Design review of the part built by this model. Coordinates are the model's own, in mm. Face numbers are marked on the shaded views. A direction names the side the tool comes from. Coordinates: 2 decimals unless noted, no trailing zeros. Loops run counter-clockwise (first coordinate to the right, second up) from the corner with the lowest first, then second, coordinate; pieces in that order, holes last. Notation, with made-up numbers: (-11.5, -21) -> (1.5, -21) arc R7 cw to (1.5, -13) -> close; hole circle Ø5 at (-20, -23.75). An arc over 180 degrees is marked (long way). Use a Markdown table: item, result. Add a question column.
Q1. Draft analysis for pull direction X (two halves, no side actions). For the marked faces 1, 2 and 3, state which applies: pulls with the +X half, pulls with the -X half, needs draft (parallel to the pull), parting line crosses it, or undercut.
Q2. Clearance check with flat-ended pins moving along their axes: pin 1 Ø4 at (x, z) = (-8, 2) entering from +Y; pin 2 Ø9 at (x, z) = (8.5, 2.5) entering from -Y; pin 3 Ø3 at (x, z) = (-3.5, 0.5) entering from -Y (3 decimals); pin 4 Ø0.8 at (x, z) = (17.5, 8) entering from +Y. State where each tip first meets the part, or that it passes through.
Q3. Take a section at B-B on z = 0. Count the separate pieces of the cut face and the enclosed holes in it, plus the area to 3 significant figures.
Q4. Take a section at C-C on y = -12.5. Write out the cut boundary in (x, z).
Q5. Take a section at A-A on y = 2.5. Write out the cut boundary in (x, z) (1 decimal).
Q6. For the marked faces 4, 5 and 6, list the 3-axis set-ups (+Z, -Z, +X, -X, +Y, -Y) from which the entire face can be reached by the end or side of a thin tool; tool diameter is ignored.
Q7. For probe 1 along Z at (x, y) = (16, -19.5); probe 2 along X at (y, z) = (3.4, 0) (1 decimal); probe 3 along Z at (x, y) = (-4.5, -17), list the stretches that pass through material, from the lowest coordinate up.
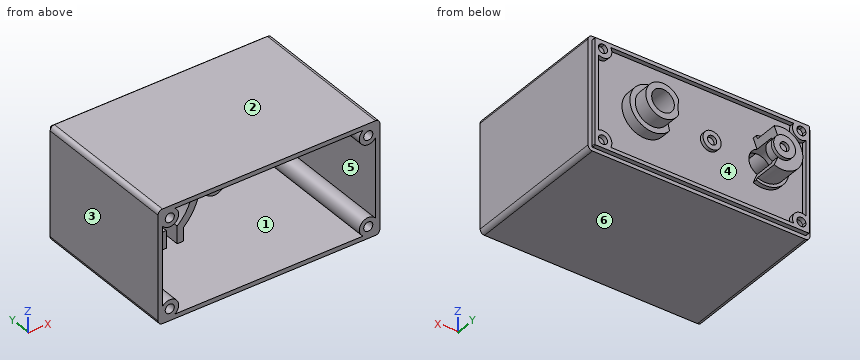
from build123d import *

# Parameters (mm, degrees)
SKETCH1_R                       = 2.3495
SKETCH1_R_2                     = 1.9812
EXTRUDE1_DEPTH                  = 1.190625
SKETCH6_R                       = 1.5875
SKETCH6_R_2                     = 0.79375
EXTRUDE3_DEPTH                  = 0.6096
SKETCH7_R                       = 3
SKETCH7_R_2                     = 1.9812
EXTRUDE4_DEPTH                  = 4.445
SKETCH16_R                      = 3.937
SKETCH16_R_2                    = 3
EXTRUDE11_DEPTH                 = 1.905
CUT_EXTRUDE1_REACH              = 24.444
SKETCH11_R                      = 7.874
SKETCH11_R_2                    = 6.604
EXTRUDE6_DEPTH                  = 4.572
SKETCH10_W                      = 37.211
SKETCH10_H                      = 18.161
EXTRUDE5_DEPTH                  = 25.90546
SKETCH13_W                      = 1.143
SKETCH13_H                      = 3.048
EXTRUDE8_DEPTH                  = 10.795
EXTRUDE9_START                  = -1.952625
SKETCH14_R                      = 0.79375
EXTRUDE9_DEPTH                  = 26.66746
SKETCH23_R                      = 0.79375
CUT_EXTRUDE2_DEPTH              = 1.190625
CUT_EXTRUDE3_REACH              = 39.594
MIRROR2_START                   = -1.952625
MIRROR2_COPY_1_SKETCH_R         = 0.79375
MIRROR2_COPY_1_DEPTH            = 26.66746
SKETCH18_W                      = 36.195
SKETCH18_H                      = 17.145
EXTRUDE12_DEPTH                 = 0.762
SKETCH19_R                      = 2.54
EXTRUDE13_DEPTH                 = 1.905
EXTRUDE14_DEPTH                 = 5.588
F_1_64_TAPPED_HOLE1_D           = 1.5113
F_1_64_TAPPED_HOLE1_DEPTH       = 5.588
F_1_64_TAPPED_HOLE1_CBORE_D     = 1.8542
F_1_64_TAPPED_HOLE1_CBORE_DEPTH = 3.7084


with BuildPart() as part:
    # Sketch1 → Extrude1 (new body)
    with BuildSketch(Plane(origin=(0, 0, 0), x_dir=(1, 0, 0), z_dir=(0, 1, 0))):
        with BuildLine():
            Line((-18.6055, 9.8425), (18.6055, 9.8425))
            ThreePointArc((18.6055, 9.8425), (19.144315367, 9.619315367), (19.3675, 9.0805))
            Line((19.3675, 9.0805), (19.3675, -9.0805))
            ThreePointArc((19.3675, -9.0805), (19.144315367, -9.619315367), (18.6055, -9.8425))
            Line((18.6055, -9.8425), (-18.6055, -9.8425))
            ThreePointArc((-18.6055, -9.8425), (-19.144315367, -9.619315367), (-19.3675, -9.0805))
            Line((-19.3675, -9.0805), (-19.3675, 9.0805))
            ThreePointArc((-19.3675, 9.0805), (-19.144315367, 9.619315367), (-18.6055, 9.8425))
        make_face()
        with Locations(Location((-11.049, 0, 0), (0, 0, 90))):
            Circle(SKETCH1_R, mode=Mode.SUBTRACT)
        with Locations(Location((9.525, 0, 0), (0, 0, 90))):
            Circle(SKETCH1_R_2, mode=Mode.SUBTRACT)
    extrude(amount=EXTRUDE1_DEPTH)

    # Sketch6 → Extrude3 (add)
    with BuildSketch(Plane(origin=(0, 1.190625, 0), x_dir=(-1, 0, 0), z_dir=(0, 1, 0))):
        with Locations(Location((1.8415, 0, 0), (0, 0, 270))):
            Circle(SKETCH6_R)
        with Locations(Location((1.8415, 0, 0), (0, 0, 90))):
            Circle(SKETCH6_R_2, mode=Mode.SUBTRACT)
    extrude(amount=EXTRUDE3_DEPTH)

    # Sketch7 → Extrude4 (add)
    with BuildSketch(Plane(origin=(0, 1.190625, 0), x_dir=(-1, 0, 0), z_dir=(0, 1, 0))):
        with Locations(Location((-9.525, 0, 0), (0, 0, 270))):
            Circle(SKETCH7_R)
        with Locations(Location((-9.525, 0, 0), (0, 0, 270))):
            Circle(SKETCH7_R_2, mode=Mode.SUBTRACT)
    extrude(amount=EXTRUDE4_DEPTH)

    # Sketch16 → Extrude11 (add)
    with BuildSketch(Plane(origin=(0, 1.190625, 0), x_dir=(-1, 0, 0), z_dir=(0, 1, 0))):
        with Locations(Location((-9.525, 0, 0), (0, 0, 270))):
            Circle(SKETCH16_R)
        with Locations(Location((-9.525, 0, 0), (0, 0, 90))):
            Circle(SKETCH16_R_2, mode=Mode.SUBTRACT)
    extrude(amount=EXTRUDE11_DEPTH)

    # Cut-Extrude1: up to this face of the body (flat: up to its plane)
    cut_extrude1_end = Plane(part.part.faces().sort_by_distance((0, 1.190625, -9.408000351))[0])
    # Sketch17 → Cut-Extrude1 (cut, up to the picked face)
    with BuildSketch(Plane(origin=(0, 5.635625, 0), x_dir=(-1, 0, 0), z_dir=(0, 1, 0)), mode=Mode.PRIVATE) as cut_extrude1_sk1:
        with BuildLine():
            ThreePointArc((-6.516949302, 2.54), (-6.894361419, 0), (-6.516949302, -2.54))
            ThreePointArc((-6.516949302, -2.54), (-5.588, 0), (-6.516949302, 2.54))
        make_face()
    cut_extrude1_tool1 = split(extrude(cut_extrude1_sk1.sketch, amount=-CUT_EXTRUDE1_REACH, mode=Mode.PRIVATE), bisect_by=cut_extrude1_end, keep=Keep.BOTH, mode=Mode.PRIVATE)
    add(cut_extrude1_tool1.solids().sort_by(Axis((6.291228, 5.635625, 0), (0, -1, 0)))[0], mode=Mode.SUBTRACT)

    # Sketch11 → Extrude6 (add)
    with BuildSketch(Plane.XZ):
        with Locations(Location((9.525, 0, 0), (0, 0, 270))):
            Circle(SKETCH11_R)
        with Locations(Location((9.525, 0, 0), (0, 0, 270))):
            Circle(SKETCH11_R_2, mode=Mode.SUBTRACT)
    extrude(amount=EXTRUDE6_DEPTH)

    # Sketch10 → Extrude5 (add)
    with BuildSketch(Plane.XZ.offset(-1.190625)):
        with BuildLine():
            Line((-19.3675, 9.0805), (-19.3675, -9.0805))
            ThreePointArc((-19.3675, -9.0805), (-19.144315367, -9.619315367), (-18.6055, -9.8425))
            Line((-18.6055, -9.8425), (18.6055, -9.8425))
            ThreePointArc((18.6055, -9.8425), (19.144315367, -9.619315367), (19.3675, -9.0805))
            Line((19.3675, -9.0805), (19.3675, 9.0805))
            ThreePointArc((19.3675, 9.0805), (19.144315367, 9.619315367), (18.6055, 9.8425))
            Line((18.6055, 9.8425), (-18.6055, 9.8425))
            ThreePointArc((-18.6055, 9.8425), (-19.144315367, 9.619315367), (-19.3675, 9.0805))
        make_face()
        Rectangle(SKETCH10_W, SKETCH10_H, mode=Mode.SUBTRACT)
    extrude(amount=EXTRUDE5_DEPTH)

    # Sketch13 → Extrude8 (add)
    with BuildSketch(Plane.XZ):
        with BuildLine():
            Line((-5.9055, 6.0325), (-5.9055, 9.0805))
            Line((-5.9055, 9.0805), (-4.7625, 9.0805))
            Line((-4.7625, 9.0805), (-4.7625, 6.713831938))
            ThreePointArc((-4.7625, 6.713831938), (-1.851412189, 0), (-4.7625, -6.713831938))
            Line((-4.7625, -6.713831938), (-4.7625, -9.0805))
            Line((-4.7625, -9.0805), (-5.9055, -9.0805))
            Line((-5.9055, -9.0805), (-5.9055, -6.0325))
            ThreePointArc((-5.9055, -6.0325), (-3.121412189, 0), (-5.9055, 6.0325))
        make_face()
        with Locations((-8.382, 7.5565)):
            Rectangle(SKETCH13_W, SKETCH13_H)
        with Locations((-13.335, 7.5565)):
            Rectangle(SKETCH13_W, SKETCH13_H)
        with Locations((-13.335, -7.5565)):
            Rectangle(SKETCH13_W, SKETCH13_H)
        with Locations((-8.382, -7.5565)):
            Rectangle(SKETCH13_W, SKETCH13_H)
    extrude(amount=EXTRUDE8_DEPTH)

    # Sketch14 → Extrude9 (add)
    with BuildSketch(Plane.XZ.offset(EXTRUDE9_START)):
        with BuildLine():
            Line((-18.6055, -9.0805), (-18.6055, -6.911913297))
            ThreePointArc((-18.6055, -6.911913297), (-16.235418625, -6.710418625), (-16.436913297, -9.0805))
            Line((-16.436913297, -9.0805), (-18.6055, -9.0805))
        make_face()
        with Locations(Location((-17.3355, -7.8105, 0), (0, 0, 270))):
            Circle(SKETCH14_R, mode=Mode.SUBTRACT)
    extrude9 = extrude(amount=EXTRUDE9_DEPTH)

    # Sketch23 → Cut-Extrude2 (cut)
    with BuildSketch(Plane(origin=(0, 1.190625, 0), x_dir=(-1, 0, 0), z_dir=(0, 1, 0))):
        with Locations(Location((17.3355, -7.8105, 0), (0, 0, 270))):
            Circle(SKETCH23_R)
    extrude(amount=-CUT_EXTRUDE2_DEPTH, mode=Mode.SUBTRACT)

    # Sketch9 → Revolve1 (revolve)
    with BuildSketch(Plane.XY, mode=Mode.PRIVATE) as revolve1_sk:
        Polygon((-12.954, 5.965825), (-12.954, 6.550025), (-11.84275, 6.550025), (-11.84275, 5.965825), (-11.049, 5.965825), (-11.049, 4.645025), (-13.3985, 4.645025), (-13.3985, 1.190625), (-15.1765, 1.190625), (-15.1765, 1.952625), (-14.6685, 1.952625), (-14.6685, 5.965825), align=None)
    revolve(revolve1_sk.sketch.rotate(Axis((-11.049, 0, 0), (0, 1, 0)), 270), axis=Axis((-11.049, 0, 0), (0, 1, 0)))

    # Cut-Extrude3: up to this face of the body (flat: up to its plane)
    cut_extrude3_end = Plane(part.part.faces().sort_by_distance((-1.8415, 1.190625, 0))[0])
    # Sketch24 → Cut-Extrude3 (cut, up to the picked face)
    with BuildSketch(Plane(origin=(0, 5.965825, 0), x_dir=(-1, 0, 0), z_dir=(0, 1, 0)), mode=Mode.PRIVATE) as cut_extrude3_sk1:
        with BuildLine():
            Line((10.316307692, 1.758461538), (9.4615, 3.81))
            ThreePointArc((9.4615, 3.81), (6.9215, 0), (9.4615, -3.81))
            Line((9.4615, -3.81), (10.316307692, -1.758461538))
            ThreePointArc((10.316307692, -1.758461538), (9.144, 0), (10.316307692, 1.758461538))
        make_face()
    cut_extrude3_tool1 = split(extrude(cut_extrude3_sk1.sketch, amount=-CUT_EXTRUDE3_REACH, mode=Mode.PRIVATE), bisect_by=cut_extrude3_end, keep=Keep.BOTH, mode=Mode.PRIVATE)
    add(cut_extrude3_tool1.solids().sort_by(Axis((-8.574349, 5.965825, 0), (0, -1, 0)))[0], mode=Mode.SUBTRACT)

    # Mirror1: Extrude9 across plane
    add(extrude9.mirror(Plane(origin=(0, 0, 0), x_dir=(0, 0, 1), z_dir=(1, 0, 0))))

    # Mirror2: Extrude9 across plane
    add(extrude9.mirror(Plane.XY))

    # Mirror2 copy 1 sketch → Mirror2 copy 1 (add)
    with BuildSketch(Plane(origin=(0, 0, 0), x_dir=(-1, 0, 0), z_dir=(0, -1, 0)).offset(MIRROR2_START)):
        with BuildLine():
            Line((-18.6055, -9.0805), (-18.6055, -6.911913297))
            ThreePointArc((-18.6055, -6.911913297), (-16.235418625, -6.710418625), (-16.436913297, -9.0805))
            Line((-16.436913297, -9.0805), (-18.6055, -9.0805))
        make_face()
        with Locations(Location((-17.3355, -7.8105, 0), (0, 0, 270))):
            Circle(MIRROR2_COPY_1_SKETCH_R, mode=Mode.SUBTRACT)
    extrude(amount=MIRROR2_COPY_1_DEPTH)

    # Sketch18 → Extrude12 (add)
    with BuildSketch(Plane(origin=(0, 1.952625, 0), x_dir=(-1, 0, 0), z_dir=(0, 1, 0))):
        with BuildLine():
            Line((18.6055, 9.2075), (-18.6055, 9.2075))
            ThreePointArc((-18.6055, 9.2075), (-18.695302561, 9.170302561), (-18.7325, 9.0805))
            Line((-18.7325, 9.0805), (-18.7325, -9.0805))
            ThreePointArc((-18.7325, -9.0805), (-18.695302561, -9.170302561), (-18.6055, -9.2075))
            Line((-18.6055, -9.2075), (18.6055, -9.2075))
            ThreePointArc((18.6055, -9.2075), (18.695302561, -9.170302561), (18.7325, -9.0805))
            Line((18.7325, -9.0805), (18.7325, 9.0805))
            ThreePointArc((18.7325, 9.0805), (18.695302561, 9.170302561), (18.6055, 9.2075))
        make_face()
        Rectangle(SKETCH18_W, SKETCH18_H, mode=Mode.SUBTRACT)
    extrude(amount=-EXTRUDE12_DEPTH)

    # Sketch19 → Extrude13 (add)
    with BuildSketch(Plane.XZ):
        with BuildLine():
            Line((11.557, -3.222898695), (11.557, -6.283612973))
            ThreePointArc((11.557, -6.283612973), (11.178939296, -6.393535861), (10.795, -6.480734218))
            Line((10.795, -6.480734218), (10.795, -3.592102448))
            ThreePointArc((10.795, -3.592102448), (9.525, -3.81), (8.255, -3.592102448))
            Line((8.255, -3.592102448), (8.255, -6.480734218))
            ThreePointArc((8.255, -6.480734218), (7.871060704, -6.393535861), (7.493, -6.283612973))
            Line((7.493, -6.283612973), (7.493, -3.222898695))
            ThreePointArc((7.493, -3.222898695), (9.525, 3.81), (11.557, -3.222898695))
        make_face()
        with Locations(Location((9.525, 0, 0), (0, 0, 90))):
            Circle(SKETCH19_R, mode=Mode.SUBTRACT)
    extrude(amount=EXTRUDE13_DEPTH)

    # Sketch20 → Extrude14 (add)
    with BuildSketch(Plane.XZ):
        with BuildLine():
            ThreePointArc((4.320531036, -4.065257532), (3.147336001, -7.413112903), (6.282470752, -5.753157401))
            ThreePointArc((6.282470752, -5.753157401), (5.218006131, -5.006258065), (4.320531036, -4.065257532))
        make_face()
    extrude(amount=EXTRUDE14_DEPTH)

    # 1-64 Tapped Hole1
    with Locations(Plane(origin=(4.389738079, -5.588, -5.969), x_dir=(0, 0, -1), z_dir=(0, -1, 0))):
        with Locations((0, 0)):
            CounterBoreHole(F_1_64_TAPPED_HOLE1_D / 2, F_1_64_TAPPED_HOLE1_CBORE_D / 2, F_1_64_TAPPED_HOLE1_CBORE_DEPTH, depth=F_1_64_TAPPED_HOLE1_DEPTH)


solid = part.part
Answer list:
| question | item | result |
|---|---|---|
| 1 | face 1 | undercut |
| 1 | face 2 | needs draft |
| 1 | face 3 | pulls with the -X half |
| 2 | pin 1 | y = 6.55 |
| 2 | pin 2 | y = -4.57 |
| 2 | pin 3 | y = -10.795 |
| 2 | pin 4 | y = 1.19 |
| 3 | separate pieces | 3 |
| 3 | enclosed holes | 0 |
| 3 | area | 128 mm² |
| 4 | outline | (-19.37, -9.08) arc R0.76 ccw to (-18.61, -9.84) -> (18.61, -9.84) arc R0.76 ccw to (19.37, -9.08) -> (19.37, 9.08) arc R0.76 ccw to (18.61, 9.84) -> (-18.61, 9.84) arc R0.76 ccw to (-19.37, 9.08) -> close; hole (-18.61, -6.91) arc R1.56 cw (long way) to (-16.44, -9.08) -> (16.44, -9.08) arc R1.56 cw (long way) to (18.61, -6.91) -> (18.61, 6.91) arc R1.56 cw (long way) to (16.44, 9.08) -> (-16.44, 9.08) arc R1.56 cw (long way) to (-18.61, 6.91) -> close; hole circle Ø1.59 at (-17.34, -7.81); hole circle Ø1.59 at (-17.34, 7.81); hole circle Ø1.59 at (17.34, -7.81); hole circle Ø1.59 at (17.34, 7.81) |
| 5 | outline | (-10.1, -2.2) arc R2.3 cw (long way) to (-10.1, 2.2) -> (-9.7, 3.3) arc R3.6 ccw (long way) to (-9.7, -3.3) -> close; (6.5, -2.5) arc R3.9 ccw (long way) to (6.5, 2.5) arc R8.7 cw to start; hole circle Ø4 at (9.5, 0) |
| 6 | face 4 | +Y |
| 6 | face 5 | -Y |
| 6 | face 6 | -Z, +X, -X, +Y, -Y |
| 7 | probe 1 | -9.84 to -9.08, -8.61 to -7.01, 7.01 to 8.61, 9.08 to 9.84 |
| 7 | probe 2 | -14.7 to -13.4, 6.9 to 7.5, 11.5 to 12.5 |
| 7 | probe 3 | -9.84 to -9.08, 9.08 to 9.84 |
